Source: CAD feature listing. Evaluate the final solid. Frame: model axes, mm. A direction names the side the tool comes from. Round coordinates to 2 decimals unless told otherwise and drop trailing zeros. Order: outer loops, then holes, each group sorted by start corner. A loop starts at its lowest first (then second) coordinate and runs counter-clockwise, first axis right, second up. Notation, with made-up numbers: (-34.75, 86.25) -> (21.25, 86.25) arc R16 ccw to (21.25, 109.25) -> close; hole circle Ø2 at (1, -19.5). An arc over 180 degrees is marked (long way). Write item = value, one per line. Start each with the question number.
(1) Contact query for flat-ended pins moving along their axis: pin 1 Ø3 at (x, y) = (0, 0) entering from +Z; pin 2 Ø1.5 at (y, z) = (-0.5, 9.5) entering from +X; pin 3 Ø2 at (x, y) = (-1.5, 7) entering from +Z; pin 4 Ø3 at (x, z) = (-6, 12.5) entering from -Y. Output: stop coordinate, or through.
(2) Reachability of faces 1 (the face through (-3.955, -5.158, 11.93)), 2 (the face through (0, 3, 0)) from +Z, -Z, +X, -X, +Y, -Y: full face, straight path, thin tool, end or side. Return the list, or none.
(3) Ray query, line 1 (X direction, y = 0, z = 13.5); line 2 (X direction, y = -2.25, z = 13.25). Return the intervals inside material, ascending.
(4) Cut plane D-D on z = 7.5. Return the cut outline in (x, y).
(5) Cut plane A-A on y = 0. Return the cut outline in (x, z), then the cut area to 3 significant figures.
(6) Draft query along X for faces 3 (the face through (-2.44, -0.54, 9.37)), 4 (the face through (8, -2, 0)), 5 (the face through (-6.62, -1.47, 6.72)). Return one class per face: released by +X, released by -X, zero draft, split by the parting line, or undercut.
(7) Cut plane C-C on z = 4. Return the cut outline in (x, y), then the cut area to 3 significant figures.
Autodesk Fusion 360 part; units mm, degrees
sketch "Base Revolution" plane through (0, 0, 0) normal (1, 0, 0) x (0, 1, 0)
  line L0 (0, 0) -> (0, 19) construction
  line L1 (0, 19) -> (2.5, 19) construction
  line L2 (2.5, 19) -> (4.5, 19)
  line L3 (4.5, 19) -> (6.5, 17)
  line L4 (6.5, 17) -> (6.5, 7)
  line L5 (6.5, 7) -> (11, 2.5)
  line L6 (11, 0) -> (2.5, 0)
  line L7 (2.5, 19) -> (2.5, 0)
  line L8 (11, 2.5) -> (11, 0)
  dimension "d2" = 12
  dimension "d3" = 19
  dimension "d4" = 4.5
  dimension "d5" = 6.5
  dimension "d6" = 2.5
  dimension "d7" = 135
  dimension "d8" = 135
  dimension "d10" = 8.5
revolve "Revolve1" add sketch "Base Revolution" angle 360 about axis through (0, 0, 0) along (0, 0, 1)
sketch "Foot cutout to reduce walking" plane through (0, 0, 0) normal (0, 1, 0) x (1, 0, 0)
  line L0 (11, -2.5) -> (-11, -2.5)
  line L1 (11, 0) -> (-11, 0)
  line L2 (2.5, 0) -> (-2.5, 0)
  line L3 (2.5, -19) -> (-2.5, -19)
  line L4 (8, 0) -> (7, -1)
  line L5 (7, -1) -> (6, 0)
  dimension "d11" = 3
  dimension "d14" = 2
revolve "Revolve2" cut sketch "Foot cutout to reduce walking" angle 360 about axis through (0, 0, 1.75) along (0, 0, 1)
equation "d4 = ( 9 / 2 ) * 1 mm"
equation "d5 = ( 13 / 2 ) * 1 mm"
equation "d6 = ( 5 / 2 ) * 1 mm"
equation "d10 = ( 17 / 2 ) * 1 mm"
Evaluation:
q1.pin_1 = through
q1.pin_2 = 6.5
q1.pin_3 = 17.34
q1.pin_4 = -4.69
q2.face_1 = +Z
q2.face_2 = -Z, +X, -X, +Y, -Y
q3.line_1 = -6.5 to -2.5, 2.5 to 6.5
q3.line_2 = -6.1 to -1.09, 1.09 to 6.1
q4.outline = circle Ø13 at (0, 0); hole circle Ø5 at (0, 0)
q5.outline = (-11, 0) -> (-8, 0) -> (-7, 1) -> (-6, 0) -> (-2.5, 0) -> (-2.5, 19) -> (-4.5, 19) -> (-6.5, 17) -> (-6.5, 7) -> (-11, 2.5) -> close; (2.5, 0) -> (6, 0) -> (7, 1) -> (8, 0) -> (11, 0) -> (11, 2.5) -> (6.5, 7) -> (6.5, 17) -> (4.5, 19) -> (2.5, 19) -> close
q5.area = 189 mm^2
q6.face_3 = undercut
q6.face_4 = zero draft
q6.face_5 = split by the parting line
q7.outline = circle Ø19 at (0, 0); hole circle Ø5 at (0, 0)
q7.area = 264 mm^2
